Input: part model. Units: mm. Frame: model coordinates. Give positions to 0.01 mm unless a question says otherwise; leave off trailing zeros. Loops run counter-clockwise (first coordinate to the right, second up) from the corner with the lowest first, then second, coordinate; pieces in that order, holes last. Notation, with made-up numbers: M 62.25,36 L 114.25,36 A25 ccw 114.25,59 Z; hole C -7,-40 d9. An arc over 180 degrees is marked long. One line per item, written item: value. Start each with the question number.
(1) Ray query, line 1 along X through (y, z) = (2.75, 32.5); line 2 along X through (y, z) = (3.25, 25.5); line 3 along X through (y, z) = (5.5, -24.5). Return the intervals inside material, ascending. Write a range as from..to.
(2) Section B-B on y = 5. State how many separate pieces and enclosed holes the cut face has, plus the area to 3 significant figures.
(3) Section D-D on z = 13.5. Output: boundary loops of the cut face in (x, y).
(4) Section A-A on z = 0. Output: boundary loops of the cut face in (x, y).
(5) Pull-direction query (X, two-part tool) for faces 1 (the cylindrical face through (1.008, 1.423, 31.078)), 2 (the flat face through (-22.98, 5.97, -22.57)), 3 (the flat face through (19.784, 5.972, 10.864)); classes: released by +X, released by -X, zero draft, split by the parting line, or undercut.
(6) Section C-C on z = -25. Output: boundary loops of the cut face in (x, y), plus the area to 3 significant figures.
(7) Pin query (flat end, axial travel): P1, Ø4, axis at y = 4.5, z = -19, coming from the -X side; P2, Ø1, axis at x = -30.5, y = 3, coming from the +Z side; P3, Ø4.5, axis at x = 22.5, y = 3, coming from the -Z side. Return the tip coordinate at first contact, or that it passes through.
```python
from build123d import *

# Parameters (mm, degrees)
SKETCH1_R           = 2.15
BOSS_EXTRUDE1_DEPTH = 8
CHAMFER1_SIZE       = 4
CHAMFER1_SIZE_2     = 6.92820323
CUT_EXTRUDE1_REACH  = 62.128
SKETCH2_R           = 1.6
CUT_EXTRUDE2_REACH  = 68.128
CUT_EXTRUDE2_START  = -6
SKETCH3_R           = 3
CIRPATTERN1_COUNT   = 3


with BuildPart() as part:
    # Sketch1 → Boss-Extrude1 (new body)
    with BuildSketch(Plane(origin=(0, 0, 0), x_dir=(1, 0, 0), z_dir=(0, 1, 0))):
        Polygon((-31, 25.980762114), (-14, 25.980762114), (-7, 32.980762114), (7, 32.980762114), (14, 25.980762114), (31, 25.980762114), (38, 13.856406461), (7, -39.837168574), (-7, -39.837168574), (-38, 13.856406461), align=None)
        with Locations(Location((0, 24.5, 0), (0, 0, 270))):
            Circle(SKETCH1_R, mode=Mode.SUBTRACT)
        with Locations(Location((0, -25.5, 0), (0, 0, 270))):
            Circle(SKETCH1_R, mode=Mode.SUBTRACT)
        with Locations(Location((0, 0, 0), (0, 0, 270))):
            Circle(SKETCH1_R, mode=Mode.SUBTRACT)
    extrude(amount=BOSS_EXTRUDE1_DEPTH)

    # Chamfer1
    # the kernel refuses this chamfer: 6.92820323, 4 mm, written as the material it takes off along each edge
    with BuildSketch(Plane(origin=(46.961927941, 8, -29.378920988), x_dir=(0.05013755556391488, -0.9983227437537926, 0.028946931201335895), z_dir=(-0.49999999999999767, 0, 0.86602540378444)), Plane(origin=(1.961927941, 8, 55.359683102), x_dir=(-0.05013755556391399, -0.9983227437537926, 0.02894693120133537), z_dir=(-0.49999999999999756, 0, -0.8660254037844402))) as chamfer1_piece_1:
        Polygon((CHAMFER1_SIZE * 0.998322743754, -CHAMFER1_SIZE * 0.0578938624027), (-CHAMFER1_SIZE_2 * 0.057893862405, -CHAMFER1_SIZE_2 * 0.998322743793), (0, 0), align=None)
    extrude(amount=97.847711765, mode=Mode.SUBTRACT)
    with BuildSketch(Plane(origin=(-3.923855882, 8, -25.980762114), x_dir=(0, -0.9983227437537926, -0.05789386240267147), z_dir=(1, 0, 0))) as chamfer1_piece_2_section:
        Polygon((CHAMFER1_SIZE * 0.998322743754, -CHAMFER1_SIZE * 0.0578938624027), (-CHAMFER1_SIZE_2 * 0.057893862405, -CHAMFER1_SIZE_2 * 0.998322743793), (0, 0), align=None)
    chamfer1_piece_2 = extrude(amount=52.847711765, mode=Mode.PRIVATE)
    chamfer1_piece_2 = split(chamfer1_piece_2, bisect_by=Plane(origin=(24.400878633, 6.686948716, -15.57988348), z_dir=(0.7071067811865477, 0, -0.7071067811865475)), keep=Keep.TOP, mode=Mode.PRIVATE)
    add(chamfer1_piece_2, mode=Mode.SUBTRACT)
    with BuildSketch(Plane(origin=(-5.674080039, 8, -45.654842153), x_dir=(0.04093714269400996, -0.9983227437537926, -0.04093714269400995), z_dir=(0.7071067811865475, 0, 0.7071067811865477))) as chamfer1_piece_3_section:
        Polygon((CHAMFER1_SIZE * 0.998322743754, -CHAMFER1_SIZE * 0.0578938624027), (-CHAMFER1_SIZE_2 * 0.057893862405, -CHAMFER1_SIZE_2 * 0.998322743793), (0, 0), align=None)
    chamfer1_piece_3 = extrude(amount=45.747206701, mode=Mode.PRIVATE)
    chamfer1_piece_3 = split(chamfer1_piece_3, bisect_by=Plane(origin=(1.830005366, 6.678491599, -25.980762114), z_dir=(0, 0, -1)), keep=Keep.TOP, mode=Mode.PRIVATE)
    add(chamfer1_piece_3, mode=Mode.SUBTRACT)
    with BuildSketch(Plane(origin=(-26.674080039, 8, -13.306682074), x_dir=(-0.04093714269400995, -0.9983227437537926, -0.04093714269400996), z_dir=(0.7071067811865477, 0, -0.7071067811865474))) as chamfer1_piece_4_section:
        Polygon((CHAMFER1_SIZE * 0.998322743754, -CHAMFER1_SIZE * 0.0578938624027), (-CHAMFER1_SIZE_2 * 0.057893862405, -CHAMFER1_SIZE_2 * 0.998322743793), (0, 0), align=None)
    chamfer1_piece_4 = extrude(amount=45.747206701, mode=Mode.PRIVATE)
    chamfer1_piece_4 = split(chamfer1_piece_4, bisect_by=Plane(origin=(-1.830005366, 6.678491599, -25.980762114), z_dir=(0, 0, -1)), keep=Keep.TOP, mode=Mode.PRIVATE)
    add(chamfer1_piece_4, mode=Mode.SUBTRACT)
    with BuildSketch(Plane(origin=(-48.923855882, 8, -25.980762114), x_dir=(0, -0.9983227437537926, -0.05789386240267147), z_dir=(1, 0, 0))) as chamfer1_piece_5_section:
        Polygon((CHAMFER1_SIZE * 0.998322743754, -CHAMFER1_SIZE * 0.0578938624027), (-CHAMFER1_SIZE_2 * 0.057893862405, -CHAMFER1_SIZE_2 * 0.998322743793), (0, 0), align=None)
    chamfer1_piece_5 = extrude(amount=52.847711765, mode=Mode.PRIVATE)
    chamfer1_piece_5 = split(chamfer1_piece_5, bisect_by=Plane(origin=(-24.400878633, 6.686948716, -15.57988348), z_dir=(-0.7071067811865474, 0, -0.7071067811865477)), keep=Keep.TOP, mode=Mode.PRIVATE)
    add(chamfer1_piece_5, mode=Mode.SUBTRACT)
    with BuildSketch(Plane(origin=(-5.674080039, 8, -45.654842153), x_dir=(0.04093714269400996, -0.9983227437537926, -0.04093714269400995), z_dir=(0.7071067811865475, 0, 0.7071067811865477))) as chamfer1_piece_6a_section:
        Polygon((CHAMFER1_SIZE * 0.998322743754, -CHAMFER1_SIZE * 0.0578938624027), (-CHAMFER1_SIZE_2 * 0.057893862405, -CHAMFER1_SIZE_2 * 0.998322743793), (0, 0), align=None)
    chamfer1_piece_6a = extrude(amount=45.747206701, mode=Mode.PRIVATE)
    chamfer1_piece_6a = split(chamfer1_piece_6a, bisect_by=Plane(origin=(17.706766412, 6.766221652, -25.980762114), z_dir=(0, 0, 1)), keep=Keep.TOP, mode=Mode.PRIVATE)
    with BuildSketch(Plane(origin=(-3.923855882, 8, -25.980762114), x_dir=(0, -0.9983227437537926, -0.05789386240267147), z_dir=(1, 0, 0))) as chamfer1_piece_6b_section:
        Polygon((CHAMFER1_SIZE * 0.998322743754, -CHAMFER1_SIZE * 0.0578938624027), (-CHAMFER1_SIZE_2 * 0.057893862405, -CHAMFER1_SIZE_2 * 0.998322743793), (0, 0), align=None)
    chamfer1_piece_6b = extrude(amount=52.847711765, mode=Mode.PRIVATE)
    chamfer1_piece_6b = split(chamfer1_piece_6b, bisect_by=Plane(origin=(11.378920334, 6.766221652, -28.60184178), z_dir=(-0.7071067811865477, 0, 0.7071067811865475)), keep=Keep.TOP, mode=Mode.PRIVATE)
    chamfer1_piece_6 = chamfer1_piece_6a & chamfer1_piece_6b
    add(chamfer1_piece_6, mode=Mode.SUBTRACT)
    with BuildSketch(Plane(origin=(-48.923855882, 8, -25.980762114), x_dir=(0, -0.9983227437537926, -0.05789386240267147), z_dir=(1, 0, 0))) as chamfer1_piece_7a_section:
        Polygon((CHAMFER1_SIZE * 0.998322743754, -CHAMFER1_SIZE * 0.0578938624027), (-CHAMFER1_SIZE_2 * 0.057893862405, -CHAMFER1_SIZE_2 * 0.998322743793), (0, 0), align=None)
    chamfer1_piece_7a = extrude(amount=52.847711765, mode=Mode.PRIVATE)
    chamfer1_piece_7a = split(chamfer1_piece_7a, bisect_by=Plane(origin=(-11.378920334, 6.766221652, -28.60184178), z_dir=(0.7071067811865474, 0, 0.7071067811865477)), keep=Keep.TOP, mode=Mode.PRIVATE)
    with BuildSketch(Plane(origin=(-26.674080039, 8, -13.306682074), x_dir=(-0.04093714269400995, -0.9983227437537926, -0.04093714269400996), z_dir=(0.7071067811865477, 0, -0.7071067811865474))) as chamfer1_piece_7b_section:
        Polygon((CHAMFER1_SIZE * 0.998322743754, -CHAMFER1_SIZE * 0.0578938624027), (-CHAMFER1_SIZE_2 * 0.057893862405, -CHAMFER1_SIZE_2 * 0.998322743793), (0, 0), align=None)
    chamfer1_piece_7b = extrude(amount=45.747206701, mode=Mode.PRIVATE)
    chamfer1_piece_7b = split(chamfer1_piece_7b, bisect_by=Plane(origin=(-17.706766412, 6.766221652, -25.980762114), z_dir=(0, 0, 1)), keep=Keep.TOP, mode=Mode.PRIVATE)
    chamfer1_piece_7 = chamfer1_piece_7a & chamfer1_piece_7b
    add(chamfer1_piece_7, mode=Mode.SUBTRACT)

    # Cut-Extrude1: up to this plane
    cut_extrude1_end = Plane(origin=(0, 0, 0), z_dir=(0, -1, 0))
    # Sketch2 → Cut-Extrude1 (cut, up to the surface)
    with BuildSketch(Plane(origin=(7.125, 14.25, 4.113620668), x_dir=(0.9013878188659966, -0.41602514716892336, -0.12009611535381544), z_dir=(0.43301270189222085, 0.8660254037844383, 0.24999999999999917)), mode=Mode.PRIVATE) as cut_extrude1_sk1:
        with Locations(Location((28.428385057, 12.896779562, 0), (0, 0, 172.874983651))):
            Circle(SKETCH2_R)
    cut_extrude1_tool1 = split(extrude(cut_extrude1_sk1.sketch, amount=-CUT_EXTRUDE1_REACH, mode=Mode.PRIVATE), bisect_by=cut_extrude1_end, keep=Keep.BOTH, mode=Mode.PRIVATE)
    # Sketch2 → Cut-Extrude1 (cut, up to the surface)
    with BuildSketch(Plane(origin=(7.125, 14.25, 4.113620668), x_dir=(0.9013878188659966, -0.41602514716892336, -0.12009611535381544), z_dir=(0.43301270189222085, 0.8660254037844383, 0.24999999999999917)), mode=Mode.PRIVATE) as cut_extrude1_sk2:
        with Locations(Location((-0.970725343, -31.201886038, 0), (0, 0, 172.874983651))):
            Circle(SKETCH2_R)
    cut_extrude1_tool2 = split(extrude(cut_extrude1_sk2.sketch, amount=-CUT_EXTRUDE1_REACH, mode=Mode.PRIVATE), bisect_by=cut_extrude1_end, keep=Keep.BOTH, mode=Mode.PRIVATE)
    # Sketch2 → Cut-Extrude1 (cut, up to the surface)
    with BuildSketch(Plane(origin=(7.125, 14.25, 4.113620668), x_dir=(0.9013878188659966, -0.41602514716892336, -0.12009611535381544), z_dir=(0.43301270189222085, 0.8660254037844383, 0.24999999999999917)), mode=Mode.PRIVATE) as cut_extrude1_sk3:
        with Locations(Location((4.576276619, -22.881383094, 0), (0, 0, 172.874983651))):
            Circle(SKETCH2_R)
    cut_extrude1_tool3 = split(extrude(cut_extrude1_sk3.sketch, amount=-CUT_EXTRUDE1_REACH, mode=Mode.PRIVATE), bisect_by=cut_extrude1_end, keep=Keep.BOTH, mode=Mode.PRIVATE)
    # Sketch2 → Cut-Extrude1 (cut, up to the surface)
    with BuildSketch(Plane(origin=(7.125, 14.25, 4.113620668), x_dir=(0.9013878188659966, -0.41602514716892336, -0.12009611535381544), z_dir=(0.43301270189222085, 0.8660254037844383, 0.24999999999999917)), mode=Mode.PRIVATE) as cut_extrude1_sk4:
        with Locations(Location((22.881383094, 4.576276619, 0), (0, 0, 172.874983651))):
            Circle(SKETCH2_R)
    cut_extrude1_tool4 = split(extrude(cut_extrude1_sk4.sketch, amount=-CUT_EXTRUDE1_REACH, mode=Mode.PRIVATE), bisect_by=cut_extrude1_end, keep=Keep.BOTH, mode=Mode.PRIVATE)
    cut_extrude1 = cut_extrude1_tool1.solids().sort_by_distance((32.75, 6, -11.691343))[0] + cut_extrude1_tool2.solids().sort_by_distance((6.25, 6, 34.208003))[0] + cut_extrude1_tool3.solids().sort_by_distance((11.25, 6, 25.547749))[0] + cut_extrude1_tool4.solids().sort_by_distance((27.75, 6, -3.031089))[0]
    add(cut_extrude1, mode=Mode.SUBTRACT)

    # Sketch3 → Cut-Extrude2 (cut, up to next)
    with BuildSketch(Plane(origin=(7.125, 14.25, 4.113620668), x_dir=(0.9013878188659967, -0.41602514716892325, -0.12009611535381544), z_dir=(0.43301270189222074, 0.8660254037844383, 0.24999999999999925)).offset(CUT_EXTRUDE2_START), mode=Mode.PRIVATE) as cut_extrude2_sk1:
        with Locations((28.428385057, 12.896779562)):
            Circle(SKETCH3_R)
    cut_extrude2_tool1 = extrude(cut_extrude2_sk1.sketch, amount=-CUT_EXTRUDE2_REACH, mode=Mode.PRIVATE) & part.part
    # Sketch3 → Cut-Extrude2 (cut, up to next)
    with BuildSketch(Plane(origin=(7.125, 14.25, 4.113620668), x_dir=(0.9013878188659967, -0.41602514716892325, -0.12009611535381544), z_dir=(0.43301270189222074, 0.8660254037844383, 0.24999999999999925)).offset(CUT_EXTRUDE2_START), mode=Mode.PRIVATE) as cut_extrude2_sk2:
        with Locations((-0.970725343, -31.201886038)):
            Circle(SKETCH3_R)
    cut_extrude2_tool2 = extrude(cut_extrude2_sk2.sketch, amount=-CUT_EXTRUDE2_REACH, mode=Mode.PRIVATE) & part.part
    # Sketch3 → Cut-Extrude2 (cut, up to next)
    with BuildSketch(Plane(origin=(7.125, 14.25, 4.113620668), x_dir=(0.9013878188659967, -0.41602514716892325, -0.12009611535381544), z_dir=(0.43301270189222074, 0.8660254037844383, 0.24999999999999925)).offset(CUT_EXTRUDE2_START), mode=Mode.PRIVATE) as cut_extrude2_sk3:
        with Locations((22.881383094, 4.576276619)):
            Circle(SKETCH3_R)
    cut_extrude2_tool3 = extrude(cut_extrude2_sk3.sketch, amount=-CUT_EXTRUDE2_REACH, mode=Mode.PRIVATE) & part.part
    # Sketch3 → Cut-Extrude2 (cut, up to next)
    with BuildSketch(Plane(origin=(7.125, 14.25, 4.113620668), x_dir=(0.9013878188659967, -0.41602514716892325, -0.12009611535381544), z_dir=(0.43301270189222074, 0.8660254037844383, 0.24999999999999925)).offset(CUT_EXTRUDE2_START), mode=Mode.PRIVATE) as cut_extrude2_sk4:
        with Locations((4.576276619, -22.881383094)):
            Circle(SKETCH3_R)
    cut_extrude2_tool4 = extrude(cut_extrude2_sk4.sketch, amount=-CUT_EXTRUDE2_REACH, mode=Mode.PRIVATE) & part.part
    cut_extrude2_1 = cut_extrude2_tool1.solids().sort_by_distance((30.151924, 0.803848, -13.191343))[0]
    add(cut_extrude2_1, mode=Mode.SUBTRACT)
    cut_extrude2_2 = cut_extrude2_tool2.solids().sort_by_distance((3.651924, 0.803848, 32.708003))[0]
    add(cut_extrude2_2, mode=Mode.SUBTRACT)
    cut_extrude2_3 = cut_extrude2_tool3.solids().sort_by_distance((25.151924, 0.803848, -4.531089))[0]
    add(cut_extrude2_3, mode=Mode.SUBTRACT)
    cut_extrude2_4 = cut_extrude2_tool4.solids().sort_by_distance((8.651924, 0.803848, 24.047749))[0]
    add(cut_extrude2_4, mode=Mode.SUBTRACT)
    cut_extrude2 = cut_extrude2_1 + cut_extrude2_2 + cut_extrude2_3 + cut_extrude2_4  # Cut-Extrude2 as one shape, for the pattern or mirror that repeats it

    # CirPattern1: Cut-Extrude1, Cut-Extrude2 ×3 about axis
    cirpattern1_axis = Axis((0, 0, 0), (0, 1, 0))
    add([cut_extrude1.rotate(cirpattern1_axis, i * 360 / CIRPATTERN1_COUNT) for i in range(1, CIRPATTERN1_COUNT)], mode=Mode.SUBTRACT)
    add([cut_extrude2.rotate(cirpattern1_axis, i * 360 / CIRPATTERN1_COUNT) for i in range(1, CIRPATTERN1_COUNT)], mode=Mode.SUBTRACT)


solid = part.part
```
Output values:
1. line 1: x = -11.24..-6.1, -2.95..2.95, 6.1..11.24
1. line 2: x = -15.28..-11.56, -8.39..-2.15, 2.15..8.39, 11.56..15.28
1. line 3: x = -11.81..-2.15, 2.15..11.81
2. separate pieces: 1
2. enclosed holes: 15
2. area: 2,930 mm²
3. outline: M -22.21,0 L 22.21,0 L 22.21,4 L 14.21,8 L -14.21,8 L -22.21,4 Z
4. outline: M -30,0 L -2.15,0 L -2.15,8 L -22,8 L -30,4 Z; M 2.15,0 L 30,0 L 30,4 L 22,8 L 2.15,8 Z
5. face 1: undercut
5. face 2: zero draft
5. face 3: released by +X
6. outline: M -31.57,0 L -2.09,0 L -2.09,8 L -5.18,8 L -13.59,4.57 L -31.57,4.57 Z; M 2.09,0 L 31.57,0 L 31.57,4.57 L 13.59,4.57 L 5.18,8 L 2.09,8 Z
6. area: 319 mm²
7. P1: stops at x = -36.19
7. P2: stops at z = 0
7. P3: stops at z = -25.98
